Verification items for the finished model (mm, model axes). Face numbers are marked on the shaded views. A direction names the side the tool comes from. Round coordinates to 2 decimals unless told otherwise and drop trailing zeros. Write each loop counter-clockwise with the first axis right and the second up, starting at its lowest first coordinate (ties: lowest second). Pieces come first, ordered by that corner, then holes. Notation, with made-up numbers: M 55,53.5 L 80,53.5 A10 ccw 80,66.5 Z; hole C -39.75,-16.5 d2. An arc over 180 degrees is marked long. Answer in a Markdown table with one row per item. Add a question column.
1. Sectioned sample at C-C on z = -1.5. Record the cut outline in (x, y), plus the area to 3 significant figures.
2. Sectioned sample at B-B on x = 0. Record the cut outline in (y, z).
3. Sectioned sample at A-A on y = 0. Record the cut outline in (x, z).
4. Sectioned sample at D-D on x = -7. Record the cut outline in (y, z), plus the area to 3 significant figures.
5. Set-up check for the marked faces 1, 2 and 3: record each of +Z, -Z, +X, -X, +Y, -Y from which the full face is reachable in a straight line by a thin tool's end or side.
6. Go/stop test with flat-tipped pins: pin 1 Ø1.5 at (y, z) = (25, -2) entering from +X; pin 2 Ø6 at (x, y) = (0, 21) entering from -Z; pin 3 Ø2 at (x, z) = (-6, 3) entering from +Y; pin 4 Ø1.5 at (x, z) = (-2.5, -2) entering from +Y. Record where each tip stops, or that it passes through.
7. Material ranges on probe 1 along Y at (x, z) = (0, -0.5); probe 2 along Y at (x, z) = (1, -2.5); probe 3 along Z at (x, y) = (-4.5, 14.5), recorded low to high.
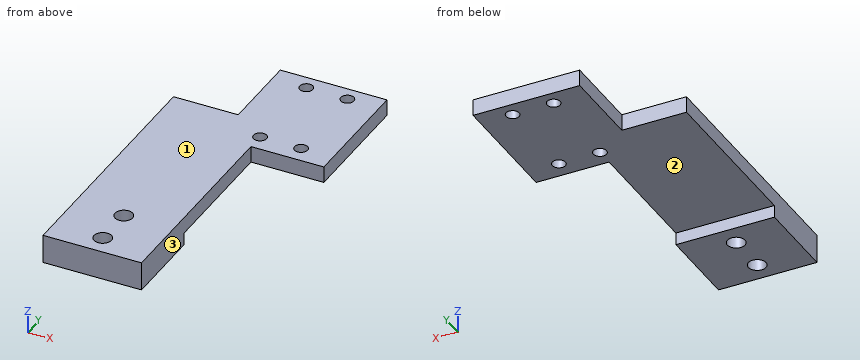
```python
from build123d import *

# Parameters (mm, degrees)
F0_R     = 1.6
F0_W     = 24
F0_H     = 20.2417488769
F0_R_2   = 2.15
F1_DEPTH = 4
F2_DEPTH = 3


# Not quite as in the source:
# - a feature names something its author has since deleted; it is built from what else it names


with BuildPart() as f1:
    # F0 (on Top) → F1 (new body)
    with BuildSketch(Plane.XY):
        Polygon((-12, 47), (-12, 5.2417488769), (12, 5.2417488769), (12, 37), (29.7651190069, 37), (29.7651190069, 67), (3.7651190069, 67), (3.7651190069, 47), align=None)
        with Locations((12, 41.3295961916)):
            Circle(F0_R, mode=Mode.SUBTRACT)
        with Locations((22, 41.3295961916)):
            Circle(F0_R, mode=Mode.SUBTRACT)
        with Locations((12, 63.3295961916)):
            Circle(F0_R, mode=Mode.SUBTRACT)
        with Locations((22, 63.3295961916)):
            Circle(F0_R, mode=Mode.SUBTRACT)
        with Locations((0, -4.8791255616)):
            Rectangle(F0_W, F0_H)
        with Locations((0, -10)):
            Circle(F0_R_2, mode=Mode.SUBTRACT)
        Circle(F0_R_2, mode=Mode.SUBTRACT)
    extrude(amount=F1_DEPTH)

    # F0 (on Top) → F2 (join)
    with BuildSketch(Plane.XY):
        with Locations((0, -4.8791255616)):
            Rectangle(F0_W, F0_H)
        with Locations((0, -10)):
            Circle(F0_R_2, mode=Mode.SUBTRACT)
        Circle(F0_R_2, mode=Mode.SUBTRACT)
    extrude(amount=-F2_DEPTH)


solid = f1.part
```
Geometry check:
| question | item | result |
|---|---|---|
| 1 | outline | M -12,-15 L 12,-15 L 12,5.24 L -12,5.24 Z; hole C 0,-10 d4.3; hole C 0,0 d4.3 |
| 1 | area | 457 mm2 |
| 2 | outline | M -15,-3 L -12.15,-3 L -12.15,4 L -15,4 Z; M -7.85,-3 L -2.15,-3 L -2.15,4 L -7.85,4 Z; M 2.15,-3 L 5.24,-3 L 5.24,0 L 47,0 L 47,4 L 2.15,4 Z |
| 3 | outline | M -12,-3 L -2.15,-3 L -2.15,4 L -12,4 Z; M 2.15,-3 L 12,-3 L 12,4 L 2.15,4 Z |
| 4 | outline | M -15,-3 L 5.24,-3 L 5.24,0 L 47,0 L 47,4 L -15,4 Z |
| 4 | area | 309 mm2 |
| 5 | face 1 | +Z, +X, -X, +Y, -Y |
| 5 | face 2 | -Z, +X, -X, +Y |
| 5 | face 3 | +Z, -Z, +X, -Y |
| 6 | pin 1 | passes through |
| 6 | pin 2 | stops at z = 0 |
| 6 | pin 3 | stops at y = 47 |
| 6 | pin 4 | stops at y = 5.24 |
| 7 | probe 1 | y = -15 to -12.15, -7.85 to -2.15, 2.15 to 5.24 |
| 7 | probe 2 | y = -15 to -11.9, -8.1 to -1.9, 1.9 to 5.24 |
| 7 | probe 3 | z = 0 to 4 |
